```python
from build123d import *

# Parameters (mm, degrees)
SKETCH1_W           = 160
SKETCH1_H           = 38.1
BOSS_EXTRUDE1_DEPTH = 6.35
SKETCH2_R           = 14.275
CUT_EXTRUDE1_DEPTH  = 7.35
SKETCH3_W           = 41
SKETCH3_H           = 21
CUT_EXTRUDE2_DEPTH  = 7.35
SKETCH4_R           = 2.75
SKETCH4_R_2         = 3.25
CUT_EXTRUDE3_DEPTH  = 7.35


with BuildPart() as part:
    # Sketch1 → Boss-Extrude1 (new body)
    with BuildSketch(Plane.XY):
        with Locations((80, -19.05)):
            Rectangle(SKETCH1_W, SKETCH1_H)
    extrude(amount=BOSS_EXTRUDE1_DEPTH)

    # Sketch2 → Cut-Extrude1 (cut, through all)
    with BuildSketch(Plane(origin=(0, 0, 0), x_dir=(-1, 0, 0), z_dir=(0, 0, -1))):
        with Locations((-140, -19.05)):
            Circle(SKETCH2_R)
    extrude(amount=-CUT_EXTRUDE1_DEPTH, mode=Mode.SUBTRACT)

    # Sketch3 → Cut-Extrude2 (cut, through all)
    with BuildSketch(Plane.XY.offset(6.35)):
        with Locations((20.5, -10.5)):
            Rectangle(SKETCH3_W, SKETCH3_H)
    extrude(amount=-CUT_EXTRUDE2_DEPTH, mode=Mode.SUBTRACT)

    # Sketch4 → Cut-Extrude3 (cut, through all)
    with BuildSketch(Plane.XY.offset(6.35)):
        with Locations((10, -29.55)):
            Circle(SKETCH4_R)
        with Locations((51, -10.5)):
            Circle(SKETCH4_R)
        with Locations((98.049601269, -29.55)):
            Circle(SKETCH4_R_2)
    extrude(amount=-CUT_EXTRUDE3_DEPTH, mode=Mode.SUBTRACT)


solid = part.part
```
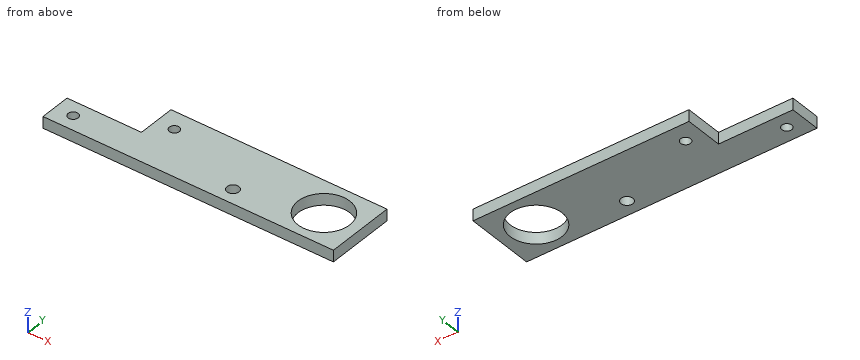
Part model, mm, in its own coordinate system. Round coordinates to 2 decimals unless told otherwise and drop trailing zeros. Order: outer loops, then holes, each group sorted by start corner. A loop starts at its lowest first (then second) coordinate and runs counter-clockwise, first axis right, second up. Notation, with made-up numbers: M 53.5,33.5 L 70.5,33.5 A6 ccw 70.5,43.5 Z; hole C -11,87 d9. An arc over 180 degrees is marked long. Answer in a Markdown table with one row per item. Add a question column.
Q1. Wall check: L1, parallel to Y at x = 51, z = 3; L2, parallel to Y at x = 140, z = 4 (3 decimals); L3, parallel to Y at x = 7, z = 5.5. Give the ranges that are in metal, low to high. Write a range as from..to.
Q2. Cut at C-C on z = 1.25. Give the cut face in (x, y) (3 decimals).
Q3. Cut at A-A on x = 140. Give the cut face in (y, z) (3 decimals).
Q4. Cut at B-B on y = -19.05. Give the cut face in (x, z) (3 decimals).
Q5. Pin check, flat tips, straight feed: pin 1 (3 mm diameter, centred on x = 27.5, z = 2, fed in from +Y); pin 2 (7 mm diameter, centred on x = 10, y = -29.55, fed in from +Z). Stop position of each tip, or through.
Q6. Cut at D-D on y = -10.5. Give the cut face in (x, z).
Established:
| question | item | result |
|---|---|---|
| 1 | L1 | y = -38.1..-13.25, -7.75..0 |
| 1 | L2 | y = -38.1..-33.325, -4.775..0 |
| 1 | L3 | y = -38.1..-21 |
| 2 | outline | M 0,-38.1 L 160,-38.1 L 160,0 L 41,0 L 41,-21 L 0,-21 Z; hole C 10,-29.55 d5.5; hole C 51,-10.5 d5.5; hole C 98.05,-29.55 d6.5; hole C 140,-19.05 d28.55 |
| 3 | outline | M -38.1,0 L -33.325,0 L -33.325,6.35 L -38.1,6.35 Z; M -4.775,0 L 0,0 L 0,6.35 L -4.775,6.35 Z |
| 4 | outline | M 41,0 L 125.725,0 L 125.725,6.35 L 41,6.35 Z; M 154.275,0 L 160,0 L 160,6.35 L 154.275,6.35 Z |
| 5 | pin 1 | stops at y = -21 |
| 5 | pin 2 | stops at z = 6.35 |
| 6 | outline | M 41,0 L 48.25,0 L 48.25,6.35 L 41,6.35 Z; M 53.75,0 L 128.57,0 L 128.57,6.35 L 53.75,6.35 Z; M 151.43,0 L 160,0 L 160,6.35 L 151.43,6.35 Z |
